Can you work these out from the drawing? Everything is in mm from the part's minimum corner. A direction names the side the tool comes from. Give positions to 0.01 mm unless a question says otherwise; leave off trailing zeros. Loops run counter-clockwise (first coordinate to the right, second up) from the corner with the lowest first, then second, coordinate; pieces in that order, holes last. Notation, with made-up numbers: (75.25, 4) - (88.25, 4) arc R30 cw to (88.25, 34) - close; hole circle Ø9 at (5, 71.25). An arc over 180 degrees is marked (long way). One line per item, written item: value. Start each with the question number.
Q1. I want a section at D-D (y = 11). Please give me the cut outline in (x, z), then the cut area to 3 significant figures.
Q2. I'm going to push flat-ended pins straight in: P1, Ø1.5, axis at x = 33.5, z = 9.5, coming from the -Y side; P2, Ø1, axis at x = 12.5, z = 8.5, coming from the -Y side; P3, Ø4, axis at y = 19, z = 7, coming from the +X side; P4, Ø8, axis at x = 23, y = 11, coming from the -Z side. Where does each tip first touch, or does it pass through?
Q3. If we mould it in two halves opening along Y, with no side actions, what happens to the marked faces 3, 4, 5 and 6? For each: released by +Y, released by -Y, zero draft, split by the parting line, or undercut.
Q4. I want a section at A-A (y = 14). Please give me the cut outline in (x, z), then the cut area to 3 significant figures.
Q5. I want a section at C-C (x = 23). Please give me the cut outline in (y, z), then the cut area to 3 significant figures.
Q6. For the marked faces 1 and 2, which set-ups out of +Z, -Z, +X, -X, +Y, -Y let a thin tool reach every point of the face, with its end or its side?
Q7. I want a section at B-B (z = 6). Please give me the cut outline in (x, y).
Q8. If I drill on line 1 (Y direction, x = 23, z = 4); line 2 (X direction, y = 3.75, z = 10.25); line 3 (X direction, y = 7, z = 3.25), over which ranges is the centre line in solid material (lowest first)? Write a range as from..to.
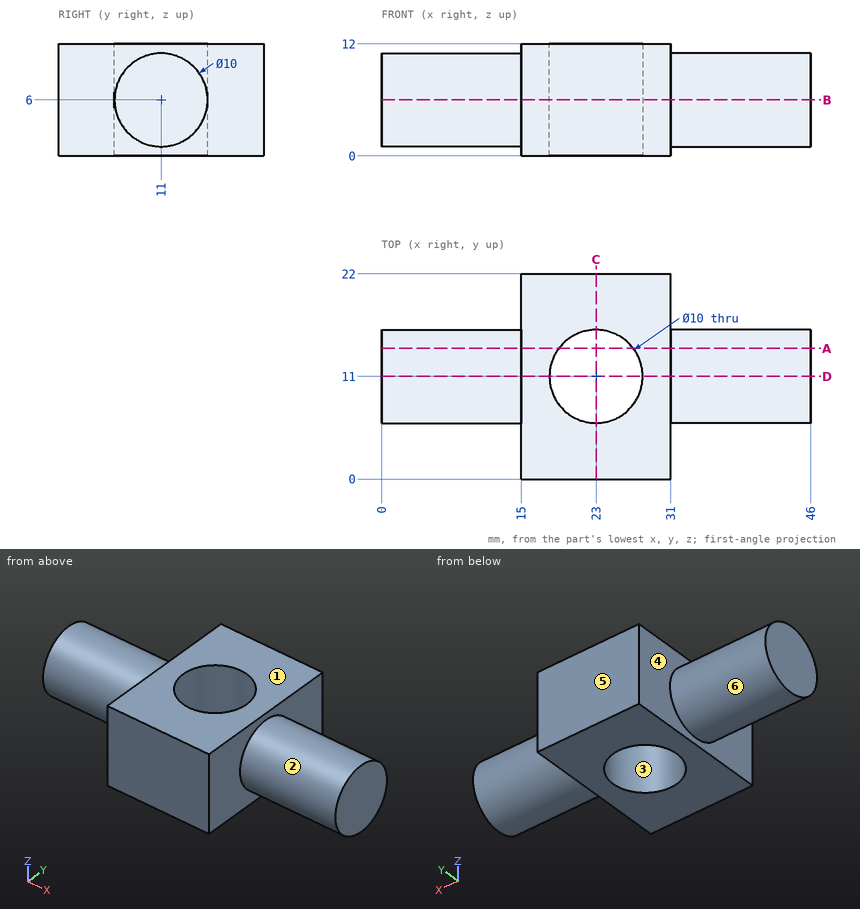
Worked answers:
1. outline: (0, 1) - (15, 1) - (15, 0) - (18, 0) - (18, 12) - (15, 12) - (15, 11) - (0, 11) - close; (28, 0) - (31, 0) - (31, 1) - (46, 1) - (46, 11) - (31, 11) - (31, 12) - (28, 12) - close
1. area: 372 mm²
2. P1: stops at y = 6.82
2. P2: stops at y = 6.42
2. P3: stops at x = 31
2. P4: passes through
3. face 3: undercut
3. face 4: zero draft
3. face 5: released by +Y
3. face 6: split by the parting line
4. outline: (0, 2) - (15, 2) - (15, 0) - (19, 0) - (19, 12) - (15, 12) - (15, 10) - (0, 10) - close; (27, 0) - (31, 0) - (31, 2) - (46, 2) - (46, 10) - (31, 10) - (31, 12) - (27, 12) - close
4. area: 336 mm²
5. outline: (0, 0) - (6, 0) - (6, 12) - (0, 12) - close; (16, 0) - (22, 0) - (22, 12) - (16, 12) - close
5. area: 144 mm²
6. face 1: +Z, +X, -X, +Y, -Y
6. face 2: +X
7. outline: (0, 6) - (15, 6) - (15, 0) - (31, 0) - (31, 6) - (46, 6) - (46, 16) - (31, 16) - (31, 22) - (15, 22) - (15, 16) - (0, 16) - close; hole circle Ø10 at (23, 11)
8. line 1: y = 0..6, 16..22
8. line 2: x = 15..31
8. line 3: x = 0..20, 26..46
